Could you check a few things on this model? Use its own coordinates, in mm. A direction names the side the tool comes from. Coordinates: 2 decimals unless noted, no trailing zeros. Write each loop counter-clockwise with the first axis right and the second up, starting at its lowest first coordinate (ties: lowest second). Pieces come first, ordered by that corner, then holes.
```python
from build123d import *
from build123d.topology import SkipClean

# Parameters (mm, degrees)
SKETCH_1_R          = 1.6
EXTRUDE_1_DEPTH     = 5
CUT_EXTRUDE_1_DEPTH = 2.5
CUT_EXTRUDE_3_DEPTH = 17.347782724
CUT_EXTRUDE_4_DEPTH = 17.911534525
SKETCH_8_W          = 6.83484861
SKETCH_8_H          = 2
CUT_EXTRUDE_5_DEPTH = 17.911534525
EXTRUDE_START       = 3
SKETCH_14_R         = 1.6
EXTRUDE_7_DEPTH     = 3
FILLET_2_R          = 2
SKETCH_15_W         = 2
SKETCH_15_H         = 4
EXTRUDE_8_DEPTH     = 5
FILLET_3_R          = 2
FILLET_4_R          = 1


# Some blends are built 0.0001 mm under size
with BuildPart() as part:
    # 草图1 → 凸台-拉伸1 (new body)
    with BuildSketch(Plane(origin=(0, 0, 0), x_dir=(1, 0, 0), z_dir=(0, 1, 0))):
        Polygon((-15, -4), (15, -4), (15, 4), (15, 6), (-15, 6), (-15, 4), align=None)
        with Locations(Location((0, 0, 0), (0, 0, 270))):
            Circle(SKETCH_1_R, mode=Mode.SUBTRACT)
    extrude(amount=EXTRUDE_1_DEPTH)

    # 草图4 → 切除-拉伸1 (cut)
    with BuildSketch(Plane.XZ):
        with BuildLine():
            Line((-13, -6), (-13, -2))
            ThreePointArc((-13, -2), (-8, 3), (-3, -2))
            Line((-3, -2), (-3, -6))
            ThreePointArc((-3, -6), (-8, -11), (-13, -6))
        make_face()
        with BuildLine():
            Line((13, -6), (13, -2))
            ThreePointArc((13, -2), (8, 3), (3, -2))
            Line((3, -2), (3, -6))
            ThreePointArc((3, -6), (8, -11), (13, -6))
        make_face()
    extrude(amount=-CUT_EXTRUDE_1_DEPTH, mode=Mode.SUBTRACT)

    # 草图6 → 切除-拉伸3 (cut, through all)
    with BuildSketch(Plane.XZ.offset(-2.5)):
        with BuildLine():
            Line((-11, -6), (-11, -2))
            ThreePointArc((-11, -2), (-8, 1), (-5, -2))
            Line((-5, -2), (-5, -6))
            ThreePointArc((-5, -6), (-8, -9), (-11, -6))
        make_face()
        with BuildLine():
            Line((11, -6), (11, -2))
            ThreePointArc((11, -2), (8, 1), (5, -2))
            Line((5, -2), (5, -6))
            ThreePointArc((5, -6), (8, -9), (11, -6))
        make_face()
    extrude(amount=-CUT_EXTRUDE_3_DEPTH, mode=Mode.SUBTRACT)

    # 草图7 → 切除-拉伸4 (cut, through all)
    with BuildSketch(Plane.XZ):
        with BuildLine():
            Line((-12.166666667, -3.236146008), (-14, -6))
            Line((-14, -6), (-13, -6))
            ThreePointArc((-13, -6), (-3.212864461, -7.443375673), (-12.166666667, -3.236146008))
        make_face()
        with BuildLine():
            Line((14, -6), (13, -6))
            ThreePointArc((13, -6), (3.212864461, -7.443375673), (12.166666667, -3.236146008))
            Line((12.166666667, -3.236146008), (14, -6))
        make_face()
    extrude(amount=-CUT_EXTRUDE_4_DEPTH, mode=Mode.SUBTRACT)

    # 草图8 → 切除-拉伸5 (cut, through all)
    with BuildSketch(Plane.XZ):
        with Locations((0, -5)):
            Rectangle(SKETCH_8_W, SKETCH_8_H)
    extrude(amount=-CUT_EXTRUDE_5_DEPTH, mode=Mode.SUBTRACT)

    # 草图14 → 凸台-拉伸7 (add)
    with SkipClean():  # the faces are left unmerged after this step: merging them gives an invalid solid
        with BuildSketch(Plane.XZ.offset(EXTRUDE_START)):
            with BuildLine():
                Line((-3, -2), (-3, -4))
                Line((-3, -4), (3, -4))
                Line((3, -4), (3, -2))
                ThreePointArc((3, -2), (3.361031331, -0.134532313), (4.391987877, 1.461538462))
                ThreePointArc((4.391987877, 1.461538462), (4.689383557, 3.088348405), (3.30958424, 4))
                Line((3.30958424, 4), (-3.30958424, 4))
                ThreePointArc((-3.30958424, 4), (-4.689383557, 3.088348405), (-4.391987877, 1.461538462))
                ThreePointArc((-4.391987877, 1.461538462), (-3.361031331, -0.134532313), (-3, -2))
            make_face()
            Circle(SKETCH_14_R, mode=Mode.SUBTRACT)
        extrude(amount=-EXTRUDE_7_DEPTH)

    # 圆角2
    # the kernel refuses this fillet: 2 mm, written as the material it takes off along each edge
    with BuildSketch(Plane(origin=(-3, -8, -4), x_dir=(0, 0, 1), z_dir=(0, 1, 0)), Plane(origin=(3, -8, -4), x_dir=(-1, 0, 0), z_dir=(0, 1, 0))) as fillet_2_piece_1:
        with BuildLine():
            CenterArc((FILLET_2_R, FILLET_2_R), FILLET_2_R, 180, 90)
            Line((0, FILLET_2_R), (0, 0))
            Line((0, 0), (FILLET_2_R, 0))
        make_face()
    extrude(amount=8, mode=Mode.SUBTRACT)
    with BuildSketch(Plane(origin=(-15, -5, 4), x_dir=(1, 0, 0), z_dir=(0, 1, 0))) as fillet_2_piece_2:
        with BuildLine():
            CenterArc((FILLET_2_R, FILLET_2_R), FILLET_2_R, 180, 90)
            Line((0, FILLET_2_R), (0, 0))
            Line((0, 0), (FILLET_2_R, 0))
        make_face()
    extrude(amount=15, mode=Mode.SUBTRACT)
    with BuildSketch(Plane(origin=(15, -5, 4), x_dir=(-1, 0, 0), z_dir=(0, 1, 0))) as fillet_2_piece_3:
        with BuildLine():
            CenterArc((FILLET_2_R, -FILLET_2_R), FILLET_2_R, 90, 90)
            Line((0, -FILLET_2_R), (0, 0))
            Line((0, 0), (FILLET_2_R, 0))
        make_face()
    extrude(amount=15, mode=Mode.SUBTRACT)
    with BuildSketch(Plane(origin=(14, -2.679237314, -6), x_dir=(1, 0, 0), z_dir=(0, 1, 0))) as fillet_2_piece_4:
        with BuildLine():
            CenterArc((1.074265007, -1.998620702), FILLET_2_R, 92.128024951, 54.314665287)
            Line((-0.59240166, -0.893079105), (0, 0))
            Line((0, 0), (1, 0))
        make_face()
    extrude(amount=10.358474629, mode=Mode.SUBTRACT)
    with BuildSketch(Plane(origin=(-14, -2.679237314, -6), x_dir=(-1, 0, 0), z_dir=(0, 1, 0))) as fillet_2_piece_5:
        with BuildLine():
            CenterArc((1.074265007, 1.998620702), FILLET_2_R, 213.557309762, 54.314665287)
            Line((-0.59240166, 0.893079105), (0, 0))
            Line((0, 0), (1, 0))
        make_face()
    extrude(amount=10.358474629, mode=Mode.SUBTRACT)
    with BuildSketch(Plane(origin=(3, 2.5, -4), x_dir=(-1, 0, 0), z_dir=(0, -1, 0))) as fillet_2_piece_6:
        with BuildLine():
            CenterArc((FILLET_2_R, -FILLET_2_R), FILLET_2_R, 90, 90)
            Line((0, -FILLET_2_R), (0, 0))
            Line((0, 0), (FILLET_2_R, 0))
        make_face()
    extrude(amount=2.5, mode=Mode.SUBTRACT)
    with BuildSketch(Plane(origin=(-3, 2.5, -4), x_dir=(1, 0, 0), z_dir=(0, -1, 0))) as fillet_2_piece_7:
        with BuildLine():
            CenterArc((FILLET_2_R, FILLET_2_R), FILLET_2_R, 180, 90)
            Line((0, FILLET_2_R), (0, 0))
            Line((0, 0), (FILLET_2_R, 0))
        make_face()
    extrude(amount=2.5, mode=Mode.SUBTRACT)

    # 草图15 → 凸台-拉伸8 (add)
    with BuildSketch(Plane.XZ):
        with Locations((16, -2)):
            Rectangle(SKETCH_15_W, SKETCH_15_H)
        with Locations((-16, -2)):
            Rectangle(SKETCH_15_W, SKETCH_15_H)
    extrude(amount=-EXTRUDE_8_DEPTH)

    # 圆角3
    fillet_3_edges = [part.edges().sort_by_distance(p)[0] for p in [
        (3.417424305, 3.75, -4),
        (-3.417424305, 3.75, -4),
        (-15, 2.5, 0),
        (15, 2.5, 0),
        (-15, 2.5, -4),
        (15, 2.5, -4),
    ]]
    fillet(fillet_3_edges, radius=FILLET_3_R - 0.0001)  # a hair under: the kernel refuses the full size

    # 圆角4
    fillet_4_edges = [part.edges().sort_by_distance(p)[0] for p in [
        (17, 2.5, 0),
        (17, 2.5, -4),
        (-17, 2.5, -4),
        (-17, 2.5, 0),
    ]]
    fillet(fillet_4_edges, radius=FILLET_4_R)


solid = part.part
```
1. I want a section at D-D on x = -8. Please give me the cut outline in (y, z).
Verdict:
outline: (0, 3) - (2.5, 3) - (2.5, 1) - (5, 1) - (5, 4) - (0, 4) - close
2. Please list where these lines run through material, in increasing order: line 1 along Z through (x, y) = (0, -0.75); line 2 along X through (y, z) = (2, 0.75); line 3 along X through (y, z) = (0.75, 0).
Verdict:
line 1: z = -4 to -1.6, 1.6 to 4
line 2: x = -15.44 to -12.18, -3.82 to -1.41, 1.41 to 3.82, 12.18 to 15.44
line 3: x = -16.56 to -12.58, -3.42 to -1.6, 1.6 to 3.42, 12.58 to 16.56
3. I want a section at B-B on z = 0.5. Please give me the cut outline in (x, y).
Verdict:
outline: (-15.68, 0) - (-12.33, 0) - (-12.33, 2.5) - (-9.66, 2.5) - (-9.66, 5) - (-15.68, 5) - close; (-6.34, 2.5) - (-3.67, 2.5) - (-3.67, -3) - (-1.52, -3) - (-1.52, 5) - (-6.34, 5) - close; (1.52, -3) - (3.67, -3) - (3.67, 2.5) - (6.34, 2.5) - (6.34, 5) - (1.52, 5) - close; (9.66, 2.5) - (12.33, 2.5) - (12.33, 0) - (15.68, 0) - (15.68, 5) - (9.66, 5) - close
4. I want a section at A-A on x = 0. Please give me the cut outline in (y, z).
Verdict:
outline: (-3, -4) - (5, -4) - (5, -1.6) - (-3, -1.6) - close; (-3, 1.6) - (5, 1.6) - (5, 4) - (-3, 4) - close
5. I want a section at C-C on y = -1.75. Please give me the cut outline in (x, z).
Verdict:
outline: (-4.39, 1.46) arc R5 cw to (-3, -2) arc R2 ccw to (-1, -4) - (1, -4) arc R2 ccw to (3, -2) arc R5 cw to (4.39, 1.46) arc R1.5 ccw to (3.31, 4) - (-3.31, 4) arc R1.5 ccw to start; hole circle Ø3.2 at (0, 0)
6. On a 3-axis mill with a long thin cutter (end or side, diameter ignored), from which of +Z, -Z, +X, -X, +Y, -Y can I reach the whole of each face in a straight line? I mean faces 1 (the face through (-12.92, 3.02, -4.37)), 2 (the face through (-14.43, 2.46, 3.4)), 3 (the face through (0, -3, 2)), 4 (the face through (9, 2.5, 1)), 5 (the face through (4.699, -1.521, 3.066)). Say none if no direction works.
Verdict:
face 1: -Z, +Y, -Y
face 2: +Z, -X, +Y, -Y
face 3: +Z, -Z, +X, -X, -Y
face 4: -Z, -Y
face 5: +X, -Y
7. If we mould it in two halves opening along X, with no side actions, what happens to faces 6 (the face through (0, 5, 2)), 7 (the face through (15.4, 2.5, 0.8)), 8 (the face through (-13, 1, -3))? For each: pulls with the +X half, pulls with the -X half, needs draft (parallel to the pull), parting line crosses it, or undercut.
Verdict:
face 6: needs draft
face 7: pulls with the +X half
face 8: undercut
8. For pin 1 (3.5 mm diameter, centred on x = 0, y = -0.5, fed in from -Z); pin 2 (1.2 mm diameter, centred on y = 1, z = -4, fed in from -X); pin 3 (3.5 mm diameter, centred on x = -10, z = 1, fed in from -Y), each with a flat end and sliding along its axis, tell me the tip position at first contact or that it passes through.
Verdict:
pin 1: stops at z = -4
pin 2: stops at x = -16.97
pin 3: stops at y = 0
